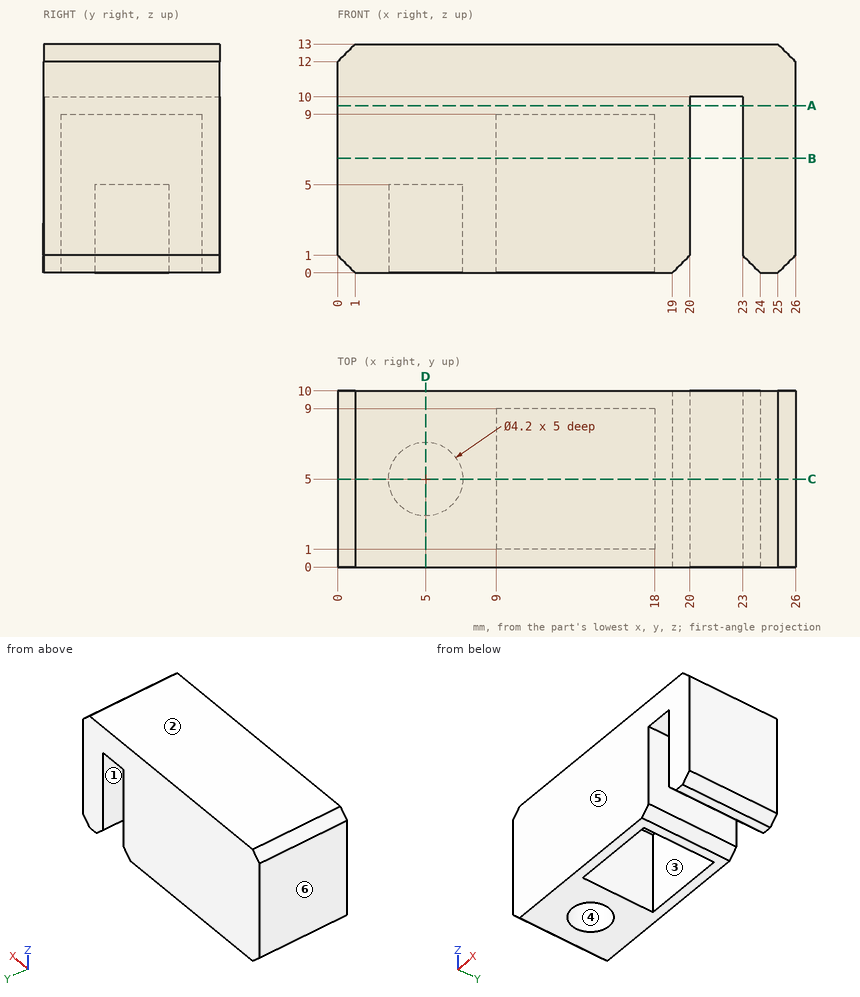
Geometry: see drawing. Coordinates: mm, zero at the bounding-box minimum. A direction names the side the tool comes from. Round coordinates to 2 decimals unless told otherwise and drop trailing zeros. Order: outer loops, then holes, each group sorted by start corner. A loop starts at its lowest first (then second) coordinate and runs counter-clockwise, first axis right, second up. Notation, with made-up numbers: (-15.5, 71.5) - (22.5, 71.5) arc R26 cw to (22.5, 88.5) - close; hole circle Ø2 at (15.5, -39). An arc over 180 degrees is marked (long way). Use a Markdown table: item, result. Add a question column.
1. Set-up query: the marked faces 1, 2 and 3. Return all of +Z, -Z, +X, -X, +Y, -Y with unobstructed straight access to the full face (end or side cutting, diameter ignored); none if empty.
2. First-contact query: pin 1 (3.5 mm diameter, centred on x = 21.5, y = 7.5, fed in from -Z); pin 2 (2.5 mm diameter, centred on x = 11.5, y = 4, fed in from -Z). Flat tips, straight axial feed; report the tip coordinate or a pass-through.
3. Section query B-B (z = 6.5). Return the cut outline in (x, y).
4. Section query C-C (y = 5). Return the cut outline in (x, z), then the cut area to 3 significant figures.
5. Line query: probe 1 along X at (y, z) = (8, 2); probe 2 along X at (y, z) = (5, 1.9); probe 3 along Y at (x, z) = (5, 3.8). Output: solid intervals per line, ascending.
6. Section query A-A (z = 9.5). Return the cut outline in (x, y), then the cut area to 3 significant figures.
7. Mould query, pull axis X, two halves, no side actions, for the marked faces 4, 5 and 6. Classes: +X half, -X half, draft (parallel to the pull), parting line (faces both ways), or undercut.
8. Section query D-D (x = 5). Return the cut outline in (y, z).
Derived:
| question | item | result |
|---|---|---|
| 1 | face 1 | -Z, +Y, -Y |
| 1 | face 2 | +Z, +X, -X, +Y, -Y |
| 1 | face 3 | -Z |
| 2 | pin 1 | z = 0.75 |
| 2 | pin 2 | z = 9 |
| 3 | outline | (0, 0) - (20, 0) - (20, 10) - (0, 10) - close; (23, 0) - (26, 0) - (26, 10) - (23, 10) - close; hole (9, 1) - (18, 1) - (18, 9) - (9, 9) - close |
| 4 | outline | (0, 1) - (1, 0) - (2.9, 0) - (2.9, 5) - (7.1, 5) - (7.1, 0) - (9, 0) - (9, 9) - (18, 9) - (18, 0) - (19, 0) - (20, 1) - (20, 10) - (23, 10) - (23, 1) - (24, 0) - (25, 0) - (26, 1) - (26, 12) - (25, 13) - (1, 13) - (0, 12) - close |
| 4 | area | 203 mm2 |
| 5 | probe 1 | 0 to 9, 18 to 20, 23 to 26 |
| 5 | probe 2 | 0 to 2.9, 7.1 to 9, 18 to 20, 23 to 26 |
| 5 | probe 3 | 0 to 2.9, 7.1 to 10 |
| 6 | outline | (0, 0) - (20, 0) - (20, 10) - (0, 10) - close; (23, 0) - (26, 0) - (26, 10) - (23, 10) - close |
| 6 | area | 230 mm2 |
| 7 | face 4 | undercut |
| 7 | face 5 | draft |
| 7 | face 6 | -X half |
| 8 | outline | (0, 0) - (2.9, 0) - (2.9, 5) - (7.1, 5) - (7.1, 0) - (10, 0) - (10, 13) - (0, 13) - close |
